Source: CAD feature listing. Evaluate the final solid. Frame: model axes, mm. Face numbers are marked on the shaded views. A direction names the side the tool comes from. Round coordinates to 2 decimals unless told otherwise and drop trailing zeros. Order: outer loops, then holes, each group sorted by start corner. A loop starts at its lowest first (then second) coordinate and runs counter-clockwise, first axis right, second up. Notation, with made-up numbers: (25.5, 13.25) - (82.5, 13.25) arc R11 cw to (82.5, 31.25) - close; hole circle Ø11 at (-14.5, 44). An arc over 180 degrees is marked (long way). Put each result on its own line as item: value. Start each with the question number.
1) Access query for the marked faces 4 and 5. Directions: +Z, -Z, +X, -X, +Y, -Y. A direction counts if a zero-diameter tool reaches every point of the face in a straight line with its end or side. Return the directions, or none.
2) Mould query, pull axis Y, two halves, no side actions, for the marked faces 1, 2 and 3. Classes: +Y half, -Y half, draft (parallel to the pull), parting line (faces both ways), or undercut.
3) Section B-B on x = 3. Output: boundary loops of the cut face in (y, z) (3 decimals).
4) Section A-A on z = 0. Output: boundary loops of the cut face in (x, y) (3 decimals).
5) Line query: probe 1 along Z at (x, y) = (3.15, 0) (3 decimals); probe 2 along Y at (x, z) = (3.5, -0.25); probe 3 along X at (y, z) = (-2, 0.25). Output: solid intervals per line, ascending. Write a range as [from, to].
6) Section D-D on x = 7.75. Output: boundary loops of the cut face in (y, z).
7) Contact query for flat-ended pins moving along their axis: P1, Ø2.5, axis at y = -0.5, z = 0, coming from the +X side; P2, Ø3, axis at y = 0, z = 0, coming from the -X side; P3, Ø1.5, axis at x = 3.5, y = 2.5, coming from the -Z side. Output: stop coordinate, or through.
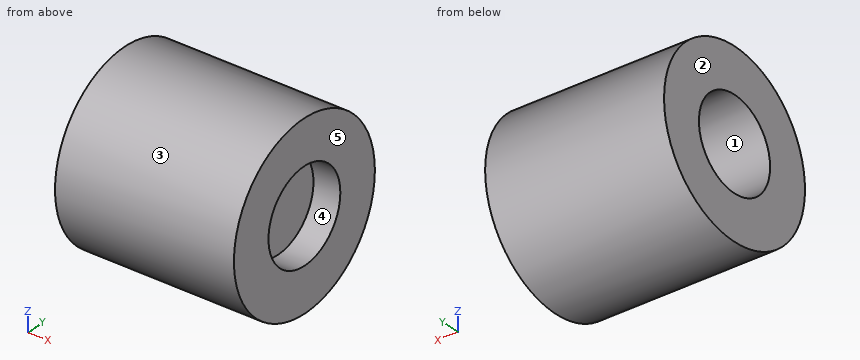
```python
from build123d import *

# Parameters (mm, degrees)
SKETCH1_R           = 5
BOSS_EXTRUDE1_DEPTH = 10
SKETCH2_R           = 2.55
CUT_EXTRUDE1_DEPTH  = 1.5
SKETCH4_R           = 2.525
CUT_EXTRUDE2_DEPTH  = 6


with BuildPart() as part:
    # Sketch1 → Boss-Extrude1 (new body)
    with BuildSketch(Plane.YZ):
        Circle(SKETCH1_R)
    extrude(amount=BOSS_EXTRUDE1_DEPTH)

    # Sketch2 → Cut-Extrude1 (cut)
    with BuildSketch(Plane.YZ.offset(10)):
        Circle(SKETCH2_R)
    extrude(amount=-CUT_EXTRUDE1_DEPTH, mode=Mode.SUBTRACT)

    # Sketch4 → Cut-Extrude2 (cut)
    with BuildSketch(Plane(origin=(0, 0, 0), x_dir=(0, -1, 0), z_dir=(-1, 0, 0))):
        Circle(SKETCH4_R)
    extrude(amount=-CUT_EXTRUDE2_DEPTH, mode=Mode.SUBTRACT)


solid = part.part
```
Answer sheet:
1. face 4: +X
1. face 5: +Z, -Z, +X, +Y, -Y
2. face 1: undercut
2. face 2: draft
2. face 3: parting line
3. outline: circle Ø10 at (0, 0); hole circle Ø5.05 at (0, 0)
4. outline: (0, -5) - (10, -5) - (10, -2.55) - (8.5, -2.55) - (8.5, 2.55) - (10, 2.55) - (10, 5) - (0, 5) - (0, 2.525) - (6, 2.525) - (6, -2.525) - (0, -2.525) - close
5. probe 1: [-5, -2.525], [2.525, 5]
5. probe 2: [-4.99, -2.51], [2.51, 4.99]
5. probe 3: [6, 8.5]
6. outline: circle Ø10 at (0, 0)
7. P1: x = 8.5
7. P2: x = 6
7. P3: z = -4.68
